Verification items for the finished model (mm, model axes). A direction names the side the tool comes from. Round coordinates to 2 decimals unless told otherwise and drop trailing zeros. Write each loop counter-clockwise with the first axis right and the second up, starting at its lowest first coordinate (ties: lowest second). Pieces come first, ordered by that corner, then holes. Notation, with made-up numbers: (76, 46) - (111, 46) arc R19 ccw to (111, 76) - close; hole circle Ø11 at (89.5, -28). An arc over 180 degrees is marked (long way). Answer as a JSON object with one key per item and string values. Group by question number.
1) Go/stop test with flat-tipped pins: pin 1 Ø12 at (y, z) = (-19.5, -28.5) entering from -X; pin 2 Ø1.7 at (x, z) = (-10, 24) entering from -Y; pin 3 Ø3.5 at (x, z) = (-21.5, 34.5) entering from -Y; pin 4 Ø1.5 at (x, z) = (-17.5, 34.5) entering from -Y. Record where each tip stops, or that it passes through.
2) Section check A-A (y = 6.5). Enter the section's corners in (x, z), then the cut area to 3 significant figures.
3) Section check B-B (y = -13). State how many separate pieces and enclosed holes the cut face has, then the cut area to 3 significant figures.
4) Mould release check, pull along X, two halves, no side actions. Record for faces 1 (the flat face through (20, 4, 47)), 2 (the flat face through (8.927, -25, -24)), 3 (the flat face through (9.405, 5, 46)), 4 (the flat face through (16, 0, 46)): +X half, -X half, draft (parallel to the pull), parting line (faces both ways), or undercut.
5) Section check D-D (z = 42). Enter the section's corners in (x, y), then the cut area to 3 significant figures.
6) Section check C-C (z = -0.5). Enter the section's corners in (x, y), then the cut area to 3 significant figures.
7) Thickness scan on line 1 (Z direction, x = -0.5, y = 9); line 2 (Y direction, x = 12, z = 25.5); line 3 (Z direction, x = -22, y = -24). Record the ranges inside material, lowest first.
8) Set-up check for faces 5 (the flat face through (-11.927, -25, 24)), 6 (the cylindrical face through (6.86, -13.03, -31.6)), 7 (the flat face through (5.927, -25, -24)): record each of +Z, -Z, +X, -X, +Y, -Y from which the full face is reachable in a straight line by a thin tool's end or side.
```python
from build123d import *

# Parameters (mm, degrees)
F1_DEPTH = 27
F4_W     = 13.767542
F4_H     = 10.494464
F5_DEPTH = 12
F2_R     = 1.5
F2_R_2   = 2.197624
F6_R     = 1.436768
F3_R     = 1.5
F7_DEPTH = 4
F8_W     = 1.44863
F8_H     = 2.5
F9_DEPTH = 20


with BuildPart() as f1:
    # F0 (on Right) → F1 (new body, symmetric)
    with BuildSketch(Plane.YZ):
        Polygon((-15, -25), (-15, -40.5), (15, -40.5), (15, -13.856175), (10, -18), (10, 18), (15, 13.856175), (15, 40.5), (-15, 40.5), (-15, 25), (-35, 25), (-35, 22.5), (-59, 22.5), (-59, -22.5), (-35, -22.5), (-35, -25), align=None)
    extrude(amount=F1_DEPTH, both=True)

    # F4 (on face) → F5 (join)
    with BuildSketch(Plane.XY.offset(40.5)):
        with Locations((16.288548, 5.247232)):
            Rectangle(F4_W, F4_H)
    extrude(amount=F5_DEPTH)

    # F2 (on face) + F6 (on face) + F3 (on face) → F7 (cut)
    with BuildSketch(Plane.XZ.offset(15)):
        with Locations((-23.745881, -35.95088)):
            Circle(F2_R)
        with Locations((-19.745881, -35.95088)):
            Circle(F2_R)
        with Locations((-15.745881, -35.95088)):
            Circle(F2_R)
        with Locations((-6.855602, -33.778694)):
            Circle(F2_R_2)
        with Locations((0.144398, -33.778694)):
            Circle(F2_R_2)
        with Locations((7.144398, -33.778694)):
            Circle(F2_R_2)
        with Locations((14.144398, -33.778694)):
            Circle(F2_R_2)
        with Locations((21.144398, -33.778694)):
            Circle(F2_R_2)
    with BuildSketch(Plane.XZ):
        with Locations((12.437331, 47.069304)):
            Circle(F6_R)
        with Locations((20.139764, 47.069304)):
            Circle(F6_R)
    with BuildSketch(Plane.XZ.offset(15)):
        with Locations((-21.891808, 34.965087)):
            Circle(F3_R)
        with Locations((-17.891808, 34.965087)):
            Circle(F3_R)
    extrude(amount=-F7_DEPTH, mode=Mode.SUBTRACT)

    # F8 (on face) → F9 (cut, through all)
    with BuildSketch(Plane.XZ.offset(35)):
        with Locations((-5.202554, 23.75)):
            Rectangle(F8_W, F8_H)
        with Locations((-8.202554, 23.75)):
            Rectangle(F8_W, F8_H)
        with Locations((-11.202554, 23.75)):
            Rectangle(F8_W, F8_H)
        with Locations((-14.202554, 23.75)):
            Rectangle(F8_W, F8_H)
        with Locations((-17.202554, 23.75)):
            Rectangle(F8_W, F8_H)
        with Locations((-20.202554, 23.75)):
            Rectangle(F8_W, F8_H)
        with Locations((5.202554, 23.75)):
            Rectangle(F8_W, F8_H)
        with Locations((8.202554, 23.75)):
            Rectangle(F8_W, F8_H)
        with Locations((11.202554, 23.75)):
            Rectangle(F8_W, F8_H)
        with Locations((14.202554, 23.75)):
            Rectangle(F8_W, F8_H)
        with Locations((17.202554, 23.75)):
            Rectangle(F8_W, F8_H)
        with Locations((20.202554, 23.75)):
            Rectangle(F8_W, F8_H)
        with Locations((-20.202554, -23.75)):
            Rectangle(F8_W, F8_H)
        with Locations((-17.202554, -23.75)):
            Rectangle(F8_W, F8_H)
        with Locations((-14.202554, -23.75)):
            Rectangle(F8_W, F8_H)
        with Locations((-11.202554, -23.75)):
            Rectangle(F8_W, F8_H)
        with Locations((-8.202554, -23.75)):
            Rectangle(F8_W, F8_H)
        with Locations((-5.202554, -23.75)):
            Rectangle(F8_W, F8_H)
        with Locations((5.202554, -23.75)):
            Rectangle(F8_W, F8_H)
        with Locations((8.202554, -23.75)):
            Rectangle(F8_W, F8_H)
        with Locations((11.202554, -23.75)):
            Rectangle(F8_W, F8_H)
        with Locations((14.202554, -23.75)):
            Rectangle(F8_W, F8_H)
        with Locations((17.202554, -23.75)):
            Rectangle(F8_W, F8_H)
        with Locations((20.202554, -23.75)):
            Rectangle(F8_W, F8_H)
    extrude(amount=-F9_DEPTH, mode=Mode.SUBTRACT)


solid = f1.part
```
Returned:
{
 "1": {"pin 1": "x = -27", "pin 2": "y = -35", "pin 3": "y = -15", "pin 4": "y = -11"},
 "2": {"outline": "(-27, -40.5) - (27, -40.5) - (27, 40.5) - (23.17, 40.5) - (23.17, 52.5) - (9.4, 52.5) - (9.4, 40.5) - (-27, 40.5) - close", "area": "4,540 mm2"},
 "3": {"separate pieces": "1", "enclosed holes": "10", "area": "4,260 mm2"},
 "4": {"face 1": "undercut", "face 2": "undercut", "face 3": "-X half", "face 4": "draft"},
 "5": {"outline": "(9.4, 0) - (23.17, 0) - (23.17, 10.49) - (9.4, 10.49) - close", "area": "144 mm2"},
 "6": {"outline": "(-27, -59) - (27, -59) - (27, 10) - (-27, 10) - close", "area": "3,730 mm2"},
 "7": {"line 1": "-40.5 to 40.5", "line 2": "-15 to 15", "line 3": "-25 to 25"},
 "8": {"face 5": "+Z, -Y", "face 6": "-Y", "face 7": "-Z, -Y"}
}
